The model under review builds one solid part; all positions refer to its coordinate system, in mm. Face numbers are marked on the shaded views. A direction names the side the tool comes from. Give positions to 0.01 mm unless a question says otherwise; leave off trailing zeros. Write each loop counter-clockwise with the first axis right and the second up, starting at its lowest first coordinate (ties: lowest second). Pieces come first, ordered by that corner, then holes. Notation, with made-up numbers: (-33.75, 8) - (-22.75, 8) arc R10 cw to (-22.75, 25) - close; hole circle Ø3 at (1.25, 71.25). An arc over 180 degrees is marked (long way). Write item = value, one per line.
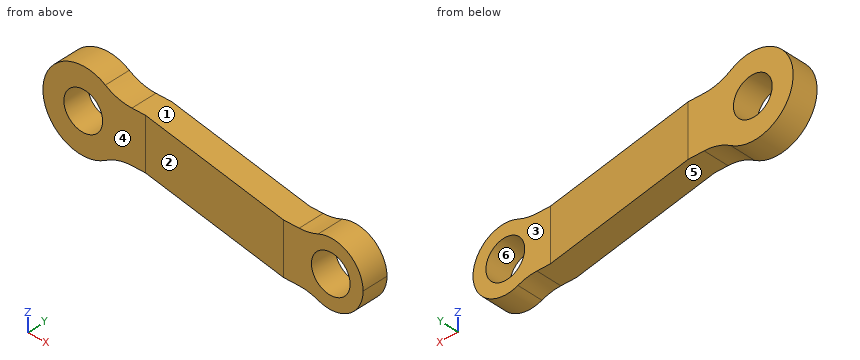
```python
from build123d import *

# Parameters (mm, degrees)
F0_R     = 6
F1_DEPTH = 25
F3_DEPTH = 12.7
F4_R     = 15
F5_R     = 15


with BuildPart() as f1:
    # F0 (on Front) → F1 (new body)
    with BuildSketch(Plane.XZ):
        with BuildLine():
            ThreePointArc((9.604686, -8), (11.753905, -4.253905), (12.5, 0))
            ThreePointArc((12.5, 0), (11.753905, 4.253905), (9.604686, 8))
            ThreePointArc((9.604686, 8), (-12.5, 0), (9.604686, -8))
        make_face()
        Circle(F0_R, mode=Mode.SUBTRACT)
        with BuildLine():
            ThreePointArc((9.604686, 8), (11.753905, 4.253905), (12.5, 0))
            ThreePointArc((12.5, 0), (11.753905, -4.253905), (9.604686, -8))
            Line((9.604686, -8), (79, -8))
            ThreePointArc((79, -8), (75, 0), (79, 8))
            Line((79, 8), (9.604686, 8))
        make_face()
        with BuildLine():
            ThreePointArc((95, 0), (89.472136, 8.944272), (79, 8))
            ThreePointArc((79, 8), (75, 0), (79, -8))
            ThreePointArc((79, -8), (89.472136, -8.944272), (95, 0))
        make_face()
        with Locations((85, 0)):
            Circle(F0_R, mode=Mode.SUBTRACT)
    extrude(amount=F1_DEPTH)

    # F2 (on Top) → F3 (intersect, symmetric)
    with BuildSketch(Plane.XY):
        Polygon((20, 0), (0, 0), (-12.5, 0), (-12.5, -8), (0, -8), (19.300091, -8), (70.341627, -17), (95, -17), (95, -9), (71.041536, -9), align=None)
    extrude(amount=F3_DEPTH, both=True, mode=Mode.INTERSECT)

    # F4
    f4_edges = [f1.edges().sort_by_distance(p)[0] for p in [
        (79, -13, 8),
    ]]
    fillet(f4_edges, radius=F4_R)

    # F5
    f5_edges = [f1.edges().sort_by_distance(p)[0] for p in [
        (9.604686, -4, 8),
        (9.604686, -4, -8),
        (79, -13, -8),
    ]]
    fillet(f5_edges, radius=F5_R)


solid = f1.part
```
1. Take a section at D-D on x = 51.5. Give the boundary of the cut face in (y, z).
Findings below:
outline = (-13.68, -8) - (-5.55, -8) - (-5.55, 8) - (-13.68, 8) - close
2. Machinability: for the marked faces 1, 2 and 3, which of the approach directions +Z, -Z, +X, -X, +Y, -Y give a long, thin tool a straight path to every point of the face, cutting with its end or side? Answer none if there is none.
Findings below:
face_1 = +Z, +Y, -Y
face_2 = +Z, -Z, -X, -Y
face_3 = +Z, -Z, +X, +Y
3. Take a section at B-B on x = 0. Give the boundary of the cut face in (y, z).
Findings below:
outline = (-8, -12.5) - (0, -12.5) - (0, -6) - (-8, -6) - close; (-8, 6) - (0, 6) - (0, 12.5) - (-8, 12.5) - close
4. Draft analysis for pull direction Z (two halves, no side actions). For the marked faces 4, 5 and 6, state which applies: +Z half, -Z half, draft (parallel to the pull), parting line (faces both ways), or undercut.
Findings below:
face_4 = draft
face_5 = -Z half
face_6 = undercut
5. Take a section at C-C on z = 7. Give the boundary of the cut face in (x, y).
Findings below:
outline = (-10.36, -8) - (19.3, -8) - (70.34, -17) - (92.14, -17) - (92.14, -9) - (71.04, -9) - (20, 0) - (-10.36, 0) - close
6. Insertion check: P1, Ø2, axis at x = 16.5, z = 7.5, coming from the -Y side; P2, Ø10, axis at y = -14, z = -8.5, coming from the +X side; P3, Ø5, axis at x = 60, z = 8, coming from the +Y side. Each pin has a flat end and moves straight along its axis. Give the tip position at first contact, or say it passes through.
Findings below:
P1 = -8
P2 = 94.37
P3 = -6.61
7. For line 1 (Z direction, x = 85, y = -11); line 2 (Z direction, x = 0, y = -2); line 3 (Y direction, x = -4.5, z = 7.25), list the stretches that pass through material, from the lowest coordinate up. Write a range as from..to.
Findings below:
line_1 = -10..-6, 6..10
line_2 = -12.5..-6, 6..12.5
line_3 = -8..0
8. Take a section at A-A on x = 85. Give the boundary of the cut face in (y, z).
Findings below:
outline = (-17, -10) - (-9, -10) - (-9, -6) - (-17, -6) - close; (-17, 6) - (-9, 6) - (-9, 10) - (-17, 10) - close
